Here's how the part is built. I have some questions about the finished solid (model axes, mm). A direction names the side the tool comes from. Round coordinates to 2 decimals unless told otherwise and drop trailing zeros. Use one line per item in the form item = value. Start each with the question number.
1. We'd pull the mould along X, two halves only. Please class faces 3 (the flat face through (-79.6, 1, 0)), 4 (the flat face through (-72, 1, 0)), 5 (the flat face through (-1, 0, -1)), 6 (the flat face through (-74.6, 1, 0)): +X half, -X half, draft (parallel to the pull), parting line (faces both ways), or undercut.
2. Will this pin go through, and if not, where does the flat tip stop? pin 1 (1.5 mm diameter, centred on x = -19.5, z = 10.5, fed in from -Y).
3. Which directions (+Z, -Z, +X, -X, +Y, -Y) give clear straight access to the entire face, cutting with the end or side of a thin tool? Please do faces 1 (the flat face through (73, 1, -7.5)), 2 (the flat face through (79.6, 1, 0)).
4. If I drill on line 1 along X through (y, z) = (0.9, 5), over which ranges is the centre line in solid material (lowest first)?
```python
from build123d import *

# Parameters (mm, degrees)
SKETCH1_W           = 159.2
SKETCH1_H           = 45
SKETCH1_W_2         = 2.6
SKETCH1_H_2         = 15
BOSS_EXTRUDE1_DEPTH = 2.5
SKETCH3_W           = 159.2
SKETCH3_H           = 10
BOSS_EXTRUDE3_DEPTH = 2.5
SKETCH4_W           = 159.2
SKETCH4_H           = 9
CUT_EXTRUDE1_DEPTH  = 3.5


with BuildPart() as part:
    # Sketch1 → Boss-Extrude1 (new body)
    with BuildSketch(Plane(origin=(0, 0, 0), x_dir=(1, 0, 0), z_dir=(0, 1, 0))):
        Rectangle(SKETCH1_W, SKETCH1_H)
        with Locations((-73.3, 0)):
            Rectangle(SKETCH1_W_2, SKETCH1_H_2, mode=Mode.SUBTRACT)
        with Locations((73.3, 0)):
            Rectangle(SKETCH1_W_2, SKETCH1_H_2, mode=Mode.SUBTRACT)
    extrude(amount=BOSS_EXTRUDE1_DEPTH)

    # Sketch3 → Boss-Extrude3 (add)
    with BuildSketch(Plane(origin=(0, 2.5, 0), x_dir=(1, 0, 0), z_dir=(0, 1, 0))):
        with Locations((0, 27.5)):
            Rectangle(SKETCH3_W, SKETCH3_H)
    extrude(amount=-BOSS_EXTRUDE3_DEPTH)

    # Sketch4 → Cut-Extrude1 (cut, through all)
    with BuildSketch(Plane(origin=(0, 2.5, 0), x_dir=(1, 0, 0), z_dir=(0, 1, 0))):
        with Locations((0, 28)):
            Rectangle(SKETCH4_W, SKETCH4_H)
    extrude(amount=-CUT_EXTRUDE1_DEPTH, mode=Mode.SUBTRACT)


solid = part.part
```
Model answer:
q1.face_3 = -X half
q1.face_4 = undercut
q1.face_5 = draft
q1.face_6 = undercut
q2.pin_1 = 0
q3.face_1 = +Y, -Y
q3.face_2 = +Z, -Z, +X, +Y, -Y
q4.line_1 = -79.6 to -74.6, -72 to 72, 74.6 to 79.6
